Source: CAD feature listing. Evaluate the final solid. Frame: model axes, mm. A direction names the side the tool comes from. Round coordinates to 2 decimals unless told otherwise and drop trailing zeros. Order: outer loops, then holes, each group sorted by start corner. A loop starts at its lowest first (then second) coordinate and runs counter-clockwise, first axis right, second up. Notation, with made-up numbers: (32.5, 87.25) - (85.5, 87.25) arc R27 cw to (85.5, 104.25) - close; hole circle Ø7 at (15.5, -0.75). An arc over 180 degrees is marked (long way). Put each result on its own line as item: value. Start each with the question number.
1) Section A-A on y = 141. Output: boundary loops of the cut face in (x, z).
2) Line query: probe 1 along X at (y, z) = (128.5, -0.5); probe 2 along Z at (x, y) = (3.5, 15.5); probe 3 along X at (y, z) = (136.5, 5.25). Output: solid intervals per line, ascending. Write a range as [from, to].
3) Contact query for flat-ended pins moving along their axis: P1, Ø2, axis at x = -1.5, y = 85.5, coming from the +Z side; P2, Ø2, axis at x = -6, y = 43.5, coming from the -Z side; P3, Ø8, axis at y = 114, z = 4.5, coming from the -X side. Output: stop coordinate, or through.
4) Access query for faces 1 (the face through (-1.808, 126.905, 8.143)), 2 (the face through (-2.286, 43.095, -7.259)). Directions: +Z, -Z, +X, -X, +Y, -Y. A direction counts if a zero-diameter tool reaches every point of the face in a straight line with its end or side. Return the directions, or none.
```python
from build123d import *

# Parameters (mm, degrees)
CROQUIS2_R              = 8.341840259
SALIENTE_EXTRUIR1_DEPTH = 85
CROQUIS3_R              = 6.858159741
SALIENTE_EXTRUIR2_DEPTH = 10


with BuildPart() as part:
    # Croquis1 → Revolución1 (revolve)
    with BuildSketch(Plane(origin=(0, 0, 0), x_dir=(0, 0, -1), z_dir=(1, 0, 0))):
        Polygon((0, 0), (6.858159741, 0), (8.341840259, 85), (0, 85), align=None)
    revolve(axis=Axis((0, 0, 0), (0, 1, 0)))

    # Croquis2 → Saliente-Extruir1 (add)
    with BuildSketch(Plane(origin=(0, 85, 0), x_dir=(1, 0, 0), z_dir=(0, 1, 0))):
        Circle(CROQUIS2_R)
    extrude(amount=SALIENTE_EXTRUIR1_DEPTH)

    # Croquis3 → Saliente-Extruir2 (add)
    with BuildSketch(Plane.XZ):
        Circle(CROQUIS3_R)
    extrude(amount=SALIENTE_EXTRUIR2_DEPTH)


solid = part.part
```
Answer sheet:
1. outline: circle Ø16.68 at (0, 0)
2. probe 1: [-8.33, 8.33]
2. probe 2: [-6.21, 6.21]
2. probe 3: [-6.48, 6.48]
3. P1: z = 8.33
3. P2: z = -5.75
3. P3: x = -8.33
4. face 1: +Y, -Y
4. face 2: -Y
